```python
from build123d import *

# Parameters (mm, degrees)
SKETCH1_R           = 14.2875
SKETCH1_R_2         = 2.54
BOSS_EXTRUDE1_DEPTH = 3.175
CUT_EXTRUDE1_DEPTH  = 162.674043733
FILLET3_R           = 6.35
SKETCH3_R           = 2.54
BOSS_EXTRUDE3_DEPTH = 3.175
SKETCH6_R           = 2.54
BOSS_EXTRUDE4_DEPTH = 3.175
FILLET2_R           = 6.35
CUT_EXTRUDE2_DEPTH  = 169.237022961
CUT_EXTRUDE3_DEPTH  = 169.237022961
CUT_EXTRUDE4_DEPTH  = 168.265702461


with BuildPart() as part:
    # Sketch1 → Boss-Extrude1 (new body)
    with BuildSketch(Plane.XY):
        with BuildLine():
            Line((-8.89, 25.4), (8.89, 25.4))
            ThreePointArc((8.89, 25.4), (17.870256121, 21.680256121), (21.59, 12.7))
            Line((21.59, 12.7), (21.59, -117.775079775))
            ThreePointArc((21.59, -117.775079775), (21.127743647, -120.388718212), (19.797058824, -122.685251408))
            Line((19.797058824, -122.685251408), (-7.952696208, -155.616779465))
            ThreePointArc((-7.952696208, -155.616779465), (-12.268297602, -157.851943494), (-16.900388255, -156.380852124))
            Line((-16.900388255, -156.380852124), (-32.439211784, -143.287061102))
            ThreePointArc((-32.439211784, -143.287061102), (-34.674375812, -138.971459708), (-33.203284443, -134.339369055))
            Line((-33.203284443, -134.339369055), (-23.382941176, -122.685251408))
            ThreePointArc((-23.382941176, -122.685251408), (-22.052256353, -120.388718212), (-21.59, -117.775079775))
            Line((-21.59, -117.775079775), (-21.59, 12.7))
            ThreePointArc((-21.59, 12.7), (-17.870256121, 21.680256121), (-8.89, 25.4))
        make_face()
        Circle(SKETCH1_R, mode=Mode.SUBTRACT)
        with Locations((0, -101.6)):
            Circle(SKETCH1_R, mode=Mode.SUBTRACT)
        with Locations((-18.532085478, -142.550133084)):
            Circle(SKETCH1_R_2, mode=Mode.SUBTRACT)
        with Locations((0, -50.8)):
            Circle(SKETCH1_R_2, mode=Mode.SUBTRACT)
    extrude(amount=BOSS_EXTRUDE1_DEPTH)

    # Sketch2 → Cut-Extrude1 (cut, through all)
    with BuildSketch(Plane.XY):
        with BuildLine():
            ThreePointArc((19.159083004, -91.647229609), (9.182340769, -50.8), (19.159083004, -9.952770391))
            ThreePointArc((19.159083004, -9.952770391), (20.973467787, -5.122670102), (21.59, 0))
            Line((21.59, 0), (27.94, 0))
            Line((27.94, 0), (27.94, -121.656687185))
            Line((27.94, -121.656687185), (-7.620284479, -163.8572221))
            Line((-7.620284479, -163.8572221), (-17.501317584, -155.874478972))
            Line((-17.501317584, -155.874478972), (16.51, -115.512152961))
            ThreePointArc((16.51, -115.512152961), (20.280273667, -109.005308906), (21.59, -101.6))
            ThreePointArc((21.59, -101.6), (20.973467787, -96.477329898), (19.159083004, -91.647229609))
        make_face()
        with BuildLine():
            Line((-21.59, -41.275), (-21.59, -60.325))
            ThreePointArc((-21.59, -60.325), (-12.065, -50.8), (-21.59, -41.275))
        make_face()
    extrude(amount=CUT_EXTRUDE1_DEPTH, mode=Mode.SUBTRACT)


with BuildPart() as cut_extrude1_piece_1:
    # of the separate pieces the step leaves, piece 1, a body of its own (cut_extrude1_pieces)
    add(part.part.solids().sort_by_distance((-8.89, 25.4, 0))[0])

    # Fillet3
    fillet3_edges = [cut_extrude1_piece_1.edges().sort_by_distance(p)[0] for p in [
        (-21.59, -41.275, 1.5875),
        (-21.59, -60.325, 1.5875),
    ]]
    fillet(fillet3_edges, radius=FILLET3_R)

    # Sketch3 → Boss-Extrude3 (add)
    with BuildSketch(Plane.XY.offset(3.175)):
        with BuildLine():
            Line((-27.351416194, -127.394768527), (-36.025496499, -137.688579))
            ThreePointArc((-36.025496499, -137.688579), (-37.217489152, -141.441859142), (-35.4063854, -144.93869507))
            Line((-35.4063854, -144.93869507), (-24.403104784, -154.210610454))
            ThreePointArc((-24.403104784, -154.210610454), (-19.771014132, -155.681701823), (-15.455412737, -153.446537795))
            Line((-15.455412737, -153.446537795), (-7.557639641, -144.073996091))
            Line((-7.557639641, -144.073996091), (-27.351416194, -127.394768527))
        make_face()
        with Locations((-18.532085478, -142.550133084)):
            Circle(SKETCH3_R, mode=Mode.SUBTRACT)
    extrude(amount=-BOSS_EXTRUDE3_DEPTH)

    # Sketch6 → Boss-Extrude4 (add)
    with BuildSketch(Plane.XY.offset(3.175)):
        Polygon((-35.4063854, -144.93869507), (-63.620410749, -121.164144113), (-51.344981666, -106.596497054), (-27.065569901, -127.055545526), align=None)
        with Locations((-52.626813855, -117.972130278)):
            Circle(SKETCH6_R, mode=Mode.SUBTRACT)
    extrude(amount=-BOSS_EXTRUDE4_DEPTH)

    # Fillet2
    fillet2_edges = [cut_extrude1_piece_1.edges().sort_by_distance(p)[0] for p in [
        (-63.620410749, -121.164144113, 1.5875),
        (-51.344981666, -106.596497054, 1.5875),
        (-27.065569901, -127.055545526, 1.5875),
    ]]
    fillet(fillet2_edges, radius=FILLET2_R)

    # Sketch7 → Cut-Extrude2 (cut, through all)
    with BuildSketch(Plane.XY.offset(3.175)):
        with BuildLine():
            Line((-21.59, 0), (-21.59, 31.75))
            Line((-21.59, 31.75), (21.59, 31.75))
            Line((21.59, 31.75), (21.59, 0))
            ThreePointArc((21.59, 0), (0, 21.59), (-21.59, 0))
        make_face()
    extrude(amount=-CUT_EXTRUDE2_DEPTH, mode=Mode.SUBTRACT)


with BuildPart() as cut_extrude1_piece_2:
    # of the separate pieces the step leaves, piece 2, a body of its own (cut_extrude1_pieces)
    add(part.part.solids().sort_by_distance((-16.900388255, -156.380852124, 0))[0])


with BuildPart() as cut_extrude3_tool:
    # Sketch10 → Cut-Extrude3 (new, through all)
    with BuildSketch(Plane.XY.offset(3.175)):
        with BuildLine():
            Line((-18.151882461, -155.32628042), (-17.361482582, -157.512020269))
            Line((-17.361482582, -157.512020269), (-14.375706423, -156.432313955))
            Line((-14.375706423, -156.432313955), (-15.455412737, -153.446537795))
            ThreePointArc((-15.455412737, -153.446537795), (-16.679911193, -154.563907595), (-18.151882461, -155.32628042))
        make_face()
    extrude(amount=-CUT_EXTRUDE3_DEPTH)


with BuildPart() as cut_extrude1_piece_1_1:
    add(cut_extrude1_piece_1.part)

    # Cut-Extrude3: cut by cut_extrude3_tool
    add(cut_extrude3_tool.part, mode=Mode.SUBTRACT)

    # Sketch12 → Cut-Extrude4 (cut, through all)
    with BuildSketch(Plane.XY.offset(3.175)):
        with BuildLine():
            Line((-21.59, -101.6), (-72.39, -101.6))
            Line((-72.39, -101.6), (-72.39, -165.1))
            Line((-72.39, -165.1), (16.51, -165.1))
            Line((16.51, -165.1), (16.51, -115.512152961))
            ThreePointArc((16.51, -115.512152961), (-7.405308906, -121.880273667), (-21.59, -101.6))
        make_face()
    extrude(amount=-CUT_EXTRUDE4_DEPTH, mode=Mode.SUBTRACT)


with BuildPart() as cut_extrude1_piece_2_1:
    add(cut_extrude1_piece_2.part)

    # Cut-Extrude3: cut by cut_extrude3_tool
    add(cut_extrude3_tool.part, mode=Mode.SUBTRACT)


solid = cut_extrude1_piece_1_1.part
```
Design review of the part built by this model. Coordinates are the model's own, in mm. A direction names the side the tool comes from. Give positions to 0.01 mm unless a question says otherwise; leave off trailing zeros. Loops run counter-clockwise (first coordinate to the right, second up) from the corner with the lowest first, then second, coordinate; pieces in that order, holes last. Notation, with made-up numbers: M 32,-20 L 78,-20 A23 cw 78,10 Z; hole C -23,19 d2. An arc over 180 degrees is marked long. Return JSON: item names as keys, results as strings. Group by question number.
Item 1: Insertion check: pin 1 Ø1 at (x, z) = (2, 1.5) entering from +Y; pin 2 Ø1 at (y, z) = (-41, 2) entering from +X; pin 3 Ø1.5 at (x, z) = (9, 1) entering from +Y. Each pin has a flat end and moves straight along its axis. Give the tip position at first contact, or say it passes through.
Item 2: We need section C-C (z = 1). Give the number of separate pieces and of enclosed holes in the cut face, and give its area (3 significant figures).
Item 3: For probe 1 along Y at (x, z) = (0, 0.7); probe 2 along Y at (x, z) = (-3, 1.85); probe 3 along Y at (x, z) = (-6.5, 1.4), list the stretches that pass through material, from the lowest coordinate up.
Item 4: Tool access review of faces 1 (the flat face through (-21.59, -18, 2)), 2 (the cylindrical face through (-20.58, -39.69, 1.61)): name each direction out of +Z, -Z, +X, -X, +Y, -Y from which nothing blocks a thin tool from reaching the whole face with its end or side.
Item 5: Mouldability with a two-part tool opening along Y and no side actions: class faces 3 (the flat face through (-4, -50, 0)), 4 (the cylindrical face through (-14.274, 0.628, 1.565)) as released by +Y, released by -Y, zero draft, split by the parting line, or undercut.
Item 6: We need section B-B (y = -50.8). Give the boundary of the cut face in (x, z) (3 decimals).
Item 7: We need section A-A (x = 0). Give the boundary of the cut face in (y, z) (1 decimal).
Item 8: We need section D-D (x = 6). Give the boundary of the cut face in (y, z) (3 decimals), and give its area (3 significant figures).
Output:
{
 "1": {"pin 1": "stops at y = 21.54", "pin 2": "stops at x = 9.78", "pin 3": "stops at y = 19.95"},
 "2": {"separate pieces": "1", "enclosed holes": "3", "area": "3,630 mm^2"},
 "3": {"probe 1": "y = -123.19 to -115.89, -87.31 to -53.34, -48.26 to -14.29, 14.29 to 21.59", "probe 2": "y = -122.98 to -115.57, -87.63 to -13.97, 13.97 to 21.38", "probe 3": "y = -122.19 to -114.32, -88.88 to -12.72, 12.72 to 20.59"},
 "4": {"face 1": "+Z, -Z, -X, +Y, -Y", "face 2": "+Z, -Z, -X"},
 "5": {"face 3": "zero draft", "face 4": "undercut"},
 "6": {"outline": "M -12.065,0 L -2.54,0 L -2.54,3.175 L -12.065,3.175 Z; M 2.54,0 L 9.182,0 L 9.182,3.175 L 2.54,3.175 Z"},
 "7": {"outline": "M -123.2,0 L -115.9,0 L -115.9,3.2 L -123.2,3.2 Z; M -87.3,0 L -53.3,0 L -53.3,3.2 L -87.3,3.2 Z; M -48.3,0 L -14.3,0 L -14.3,3.2 L -48.3,3.2 Z; M 14.3,0 L 21.6,0 L 21.6,3.2 L 14.3,3.2 Z"},
 "8": {"outline": "M -122.34,0 L -114.567,0 L -114.567,3.175 L -122.34,3.175 Z; M -88.633,0 L -12.967,0 L -12.967,3.175 L -88.633,3.175 Z; M 12.967,0 L 20.74,0 L 20.74,3.175 L 12.967,3.175 Z", "area": "290 mm^2"}
}
